Design review of the part built by this model. Coordinates are the model's own, in mm. Face numbers are marked on the shaded views. A direction names the side the tool comes from. Round coordinates to 2 decimals unless told otherwise and drop trailing zeros. Order: outer loops, then holes, each group sorted by start corner. A loop starts at its lowest first (then second) coordinate and runs counter-clockwise, first axis right, second up. Notation, with made-up numbers: M 58.25,22 L 94.25,22 A31 ccw 94.25,53 Z; hole C 43.5,80 d11. An arc over 180 degrees is marked long. Use a Markdown table: item, result. Add a question column.
(1) Take a section at D-D (x = 0). Write out the cut boundary in (y, z).
(2) Take a section at A-A (z = 20). Write out the cut boundary in (x, y).
(3) For pin 1 (2.5 mm diameter, centred on x = 10, z = 15, fed in from +Y); pin 2 (5 mm diameter, centred on x = -0.5, z = 18, fed in from -Y); pin 3 (3 mm diameter, centred on x = 10, z = 5, fed in from +Y), all flat-tipped, find the tip position at first contact; note any pin that passes through.
(4) The part is to be moulded in two halves that separate along Z. For the marked faces 1, 2, 3 and 4, say which applies: released by +Z, released by -Z, zero draft, split by the parting line, or undercut.
(5) Take a section at B-B (x = 10). Write out the cut boundary in (y, z).
(6) To check wall thickness, follow probe 1 along Z at (x, y) = (-10, 4.5); probe 2 along Y at (x, z) = (0.25, 7.5); probe 3 along Z at (x, y) = (-9.5, 9.5). State the ranges of each line that lie inside material, in increasing order. Write a range as from..to.
(7) Machinability: for the marked faces 5, 6, 7, 8 and 9, which of the approach directions +Z, -Z, +X, -X, +Y, -Y give a long, thin tool a straight path to every point of the face, cutting with its end or side? Answer none if there is none.
(8) Take a section at C-C (y = 9). Write out the cut boundary in (x, z).
```python
from build123d import *

# Parameters (mm, degrees)
BOSS_EXTRU_1_DEPTH      = 25
ESQUISSE2_R             = 6
ENL_V_MAT_EXTRU_1_DEPTH = 25
ESQUISSE3_R             = 2
ENL_V_MAT_EXTRU_2_DEPTH = 33.787192622
ESQUISSE4_W             = 10
ESQUISSE4_H             = 25
ENL_V_MAT_EXTRU_3_DEPTH = 0.5


with BuildPart() as part:
    # Esquisse1 → Boss.-Extru.1 (new body)
    with BuildSketch(Plane.XY):
        Polygon((15, 0), (-15, 0), (-15, 15), (-7, 15), (-4, 18), (4, 18), (7, 15), (15, 15), align=None)
    extrude(amount=BOSS_EXTRU_1_DEPTH)

    # Esquisse2 → Enlèv. mat.-Extru.1 (cut)
    with BuildSketch(Plane.XY.offset(25)):
        with Locations((0, 9)):
            Circle(ESQUISSE2_R)
    extrude(amount=-ENL_V_MAT_EXTRU_1_DEPTH, mode=Mode.SUBTRACT)

    # Esquisse3 → Enlèv. mat.-Extru.2 (cut, through all)
    with BuildSketch(Plane(origin=(0, 15, 0), x_dir=(1, 0, 0), z_dir=(0, 1, 0))):
        with Locations(Location((-10, -5, 0), (0, 0, 180))):
            Circle(ESQUISSE3_R)
        with Locations((10, -5)):
            Circle(ESQUISSE3_R)
        with Locations(Location((10, -20, 0), (0, 0, 180))):
            Circle(ESQUISSE3_R)
        with Locations((-10, -20)):
            Circle(ESQUISSE3_R)
    extrude(amount=-ENL_V_MAT_EXTRU_2_DEPTH, mode=Mode.SUBTRACT)

    # Esquisse4 → Enlèv. mat.-Extru.3 (cut)
    with BuildSketch(Plane.XZ):
        with Locations((0, 12.5)):
            Rectangle(ESQUISSE4_W, ESQUISSE4_H)
    extrude(amount=-ENL_V_MAT_EXTRU_3_DEPTH, mode=Mode.SUBTRACT)


solid = part.part
```
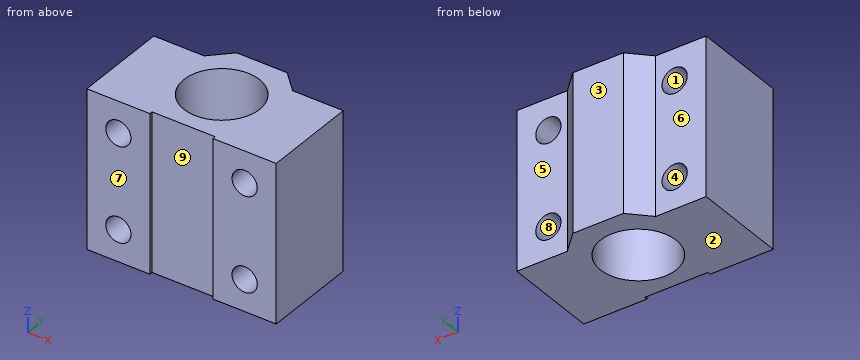
Verdict:
| question | item | result |
|---|---|---|
| 1 | outline | M 0.5,0 L 3,0 L 3,25 L 0.5,25 Z; M 15,0 L 18,0 L 18,25 L 15,25 Z |
| 2 | outline | M -15,0 L -12,0 L -12,15 L -15,15 Z; M -8,0 L -5,0 L -5,0.5 L 5,0.5 L 5,0 L 8,0 L 8,15 L 7,15 L 4,18 L -4,18 L -7,15 L -8,15 Z; M 12,0 L 15,0 L 15,15 L 12,15 Z; hole C 0,9 d12 |
| 3 | pin 1 | stops at y = 15 |
| 3 | pin 2 | stops at y = 0.5 |
| 3 | pin 3 | passes through |
| 4 | face 1 | undercut |
| 4 | face 2 | released by -Z |
| 4 | face 3 | zero draft |
| 4 | face 4 | undercut |
| 5 | outline | M 0,0 L 15,0 L 15,3 L 0,3 Z; M 0,7 L 15,7 L 15,18 L 0,18 Z; M 0,22 L 15,22 L 15,25 L 0,25 Z |
| 6 | probe 1 | z = 0..3, 7..18, 22..25 |
| 6 | probe 2 | y = 0.5..3.01, 14.99..18 |
| 6 | probe 3 | z = 0..3.06, 6.94..18.06, 21.94..25 |
| 7 | face 5 | +Z, -Z, +X, +Y |
| 7 | face 6 | +Z, -Z, -X, +Y |
| 7 | face 7 | +Z, -Z, +X, -X, -Y |
| 7 | face 8 | +Y, -Y |
| 7 | face 9 | +Z, -Z, -Y |
| 8 | outline | M -15,0 L -6,0 L -6,25 L -15,25 Z; M 6,0 L 15,0 L 15,25 L 6,25 Z; hole C -10,5 d4; hole C -10,20 d4; hole C 10,5 d4; hole C 10,20 d4 |
